from build123d import *

# Parameters (mm, degrees)
F0_R     = 3
F1_DEPTH = 1


with BuildPart() as f1:
    # F0 (on Top) → F1 (new body)
    with BuildSketch(Plane.XY):
        with BuildLine():
            ThreePointArc((14.491269, -13.784162), (18.477591, -7.653669), (19.993749, -0.5))
            Line((19.993749, -0.5), (12.443239, -0.5))
            ThreePointArc((12.443239, -0.5), (8.450707, -1.966982), (8.924937, 2.260009))
            Line((8.924937, 2.260009), (7.814871, 4.681242))
            ThreePointArc((7.814871, 4.681242), (4.591124, 7.41562), (8.445145, 9.152252))
            Line((8.445145, 9.152252), (13.784162, 14.491269))
            ThreePointArc((13.784162, 14.491269), (7.653669, 18.477591), (0.5, 19.993749))
            Line((0.5, 19.993749), (0.5, 12.443239))
            ThreePointArc((0.5, 12.443239), (2.111531, 8.655304), (-2.001884, 8.496265))
            Line((-2.001884, 8.496265), (-4.569773, 7.19161))
            ThreePointArc((-4.569773, 7.19161), (-7.726287, 4.655242), (-9.152252, 8.445145))
            Line((-9.152252, 8.445145), (-14.491269, 13.784162))
            ThreePointArc((-14.491269, 13.784162), (-18.477591, 7.653669), (-19.993749, 0.5))
            Line((-19.993749, 0.5), (-12.443239, 0.5))
            ThreePointArc((-12.443239, 0.5), (-8.418362, 1.941174), (-9.000323, -2.294146))
            Line((-9.000323, -2.294146), (-8.081482, -4.781892))
            ThreePointArc((-8.081482, -4.781892), (-4.575258, -7.273959), (-8.445145, -9.152252))
            Line((-8.445145, -9.152252), (-13.784162, -14.491269))
            ThreePointArc((-13.784162, -14.491269), (-7.653669, -18.477591), (-0.5, -19.993749))
            Line((-0.5, -19.993749), (-0.5, -12.443239))
            ThreePointArc((-0.5, -12.443239), (-1.769645, -8.227862), (2.448421, -9.488543))
            Line((2.448421, -9.488543), (4.89789, -8.310227))
            ThreePointArc((4.89789, -8.310227), (7.14589, -4.567904), (9.152252, -8.445145))
            Line((9.152252, -8.445145), (14.491269, -13.784162))
        make_face()
        Circle(F0_R, mode=Mode.SUBTRACT)
    extrude(amount=F1_DEPTH)


solid = f1.part
Geometry check sheet. Reference: the model listing, model coordinates, mm. A direction names the side the tool comes from. Give positions to 0.01 mm unless a question says otherwise; leave off trailing zeros. Write each loop counter-clockwise with the first axis right and the second up, starting at its lowest first coordinate (ties: lowest second). Pieces come first, ordered by that corner, then holes. Notation, with made-up numbers: M 4,78.25 L 11,78.25 A9 cw 11,83.25 Z; hole C 28.25,72 d1. An arc over 180 degrees is marked long. Answer as CSV lines item,"result". Start each with the question number.
Q1. Section check C-C, the plane z = 0.55. Record the cut outline in (x, y), then the cut area to 3 significant figures.
Q2. Go/stop test with a flat-tipped pin: pin 1 (0.5 mm diameter, centred on x = 18, z = 0.5, fed in from +Y). Record where the tip stops, or that it passes through.
Q3. Section check D-D, the plane x = 16. Record the cut outline in (y, z), then the cut area to 3 significant figures.
Q4. Section check A-A, the plane x = 0. Record the cut outline in (y, z).
Q5. Release check for a two-part mould opening along Y. For faces 6 (the face through (-3, -1, 1)), 7 (the face through (2.147, 8.713, 0.493)), 8 (the face through (4.582, 7.346, 0.493)), 9 (the face through (7.749, 18.438, 0.493)) record: pulls with the +Y half, pulls with the -Y half, needs draft (parallel to the pull), parting line crosses it, or undercut.
Q6. Material ranges on L1, parallel to X at y = 8, z = 0.8; L2, parallel to X at y = 6, z = 0.2; L3, parallel to Y at x = 0, z = 0.5, recorded low to high.
Q7. Tool access check on faces 1 (the face through (11.077, 11.784, 0.493)), 2 (the face through (-16.3, 0.5, 0.5)), 3 (the face through (-4.57, -7.2, 0.49)), 4 (the face through (-11.784, 11.077, 0.493)), 5 (the face through (3.656, -8.908, 0.493)). Record the directions out of +Z, -Z, +X, -X, +Y, -Y that give a thin tool (end or side, any length) a straight path to the whole face; none if there is none.
Geometry says:
1,outline,"M -19.99,0.5 L -12.44,0.5 A2.5 cw long -9,-2.29 L -8.08,-4.78 A2.5 cw long -8.45,-9.15 L -13.78,-14.49 A20 ccw -0.5,-19.99 L -0.5,-12.44 A2.5 cw long 2.45,-9.49 L 4.9,-8.31 A2.5 cw long 9.15,-8.45 L 14.49,-13.78 A20 ccw 19.99,-0.5 L 12.44,-0.5 A2.5 cw long 8.92,2.26 L 7.81,4.68 A2.5 cw long 8.45,9.15 L 13.78,14.49 A20 ccw 0.5,19.99 L 0.5,12.44 A2.5 cw long -2,8.5 L -4.57,7.19 A2.5 cw long -9.15,8.45 L -14.49,13.78 A20 ccw Z; hole C 0,0 d6"
1,area,"602 mm^2"
2,pin 1,"y = -0.5"
3,outline,"M -12,0 L -0.5,0 L -0.5,1 L -12,1 Z"
3,area,"11.5 mm^2"
4,outline,"M -7.49,0 L -3,0 L -3,1 L -7.49,1 Z; M 3,0 L 7.49,0 L 7.49,1 L 3,1 Z"
5,face 6,"needs draft"
5,face 7,"undercut"
5,face 8,"undercut"
5,face 9,"pulls with the +Y half"
6,L1,"-18.33 to -9.39, -2.98 to -1.51, 1.51 to 4.75"
6,L2,"-19.08 to -9.33, -4.81 to 4.81"
6,L3,"-7.49 to -3, 3 to 7.49"
7,face 1,"+Z, -Z, +X"
7,face 2,"+Z, -Z, -X"
7,face 3,"+Z, -Z"
7,face 4,"+Z, -Z, +Y"
7,face 5,"+Z, -Z, -Y"
